Source: CAD feature listing. Evaluate the final solid. Frame: model axes, mm. Face numbers are marked on the shaded views. A direction names the side the tool comes from. Give positions to 0.01 mm unless a question says otherwise; leave off trailing zeros. Order: outer loops, then holes, each group sorted by start corner. A loop starts at its lowest first (then second) coordinate and runs counter-clockwise, first axis right, second up. Notation, with made-up numbers: M -8.75,-6 L 36.25,-6 A23 cw 36.25,19 Z; hole C -13.75,0 d8. An arc over 180 degrees is marked long. Answer in a Markdown table with one row per item. Add a question column.
(1) Section query B-B, the plane y = 22. Return loops of the section in (x, z), plus the area to 3 significant figures.
(2) Material intervals for line 1 along Y through (x, z) = (-11, 23.5); line 2 along Z through (x, y) = (-8, 21); line 3 along X through (y, z) = (9.5, 18.75), sorted ascending.
(3) Section query D-D, the plane x = -13. Return loops of the section in (y, z), plus the area to 3 significant figures.
(4) Set-up query: the marked faces 1, 2, 3 and 4. Return all of +Z, -Z, +X, -X, +Y, -Y with unobstructed straight access to the full face (end or side cutting, diameter ignored); none if empty.
(5) Section query A-A, the plane x = 8. Return loops of the section in (y, z).
(6) Section query C-C, the plane z = 26.25. Return loops of the section in (x, y).
(7) Pin query (flat end, axial travel): P1, Ø2, axis at x = 2, y = 6.5, coming from the -Z side; P2, Ø18, axis at x = 3.5, y = 13.5, coming from the +Z side; P3, Ø3, axis at y = 6.5, z = 14, coming from the +X side; P4, Ø1, axis at y = 30.5, z = 20.5, coming from the +X side. Return the tip coordinate at first contact, or that it passes through.
from build123d import *

# Parameters (mm, degrees)
F1_DEPTH = 15
F3_DEPTH = 28
F0_W     = 23
F0_H     = 10
F4_DEPTH = 15


with BuildPart() as f1:
    # F0 (on Right) → F1 (new body, symmetric)
    with BuildSketch(Plane.YZ):
        Polygon((0, 8), (0, 0), (36, 0), (36, 20), align=None)
    extrude(amount=F1_DEPTH, both=True)

    # F2 (on face) → F3 (join)
    with BuildSketch(Plane(origin=(0, 0, 0), x_dir=(1, 0, 0), z_dir=(0, 0, -1))):
        Polygon((4.5, 0), (-4.5, 0), (-15, -36), (15, -36), align=None)
    extrude(amount=-F3_DEPTH)

    # F0 (on Right) → F4 (cut, symmetric)
    with BuildSketch(Plane.YZ):
        with Locations((11.5, 25)):
            Rectangle(F0_W, F0_H)
    extrude(amount=F4_DEPTH, both=True, mode=Mode.SUBTRACT)


solid = f1.part
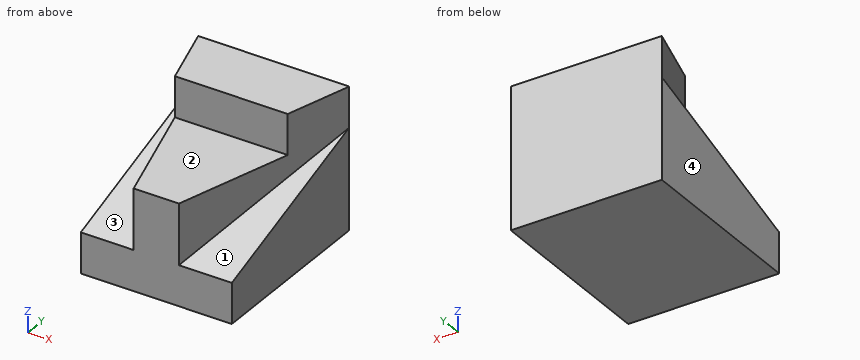
Values follow:
| question | item | result |
|---|---|---|
| 1 | outline | M -15,0 L 15,0 L 15,15.33 L 10.92,15.33 L 10.92,20 L -10.92,20 L -10.92,15.33 L -15,15.33 Z |
| 1 | area | 562 mm² |
| 2 | line 1 | y = 23 to 36 |
| 2 | line 2 | z = 0 to 20 |
| 2 | line 3 | x = -7.27 to 7.27 |
| 3 | outline | M 0,0 L 36,0 L 36,28 L 29.14,28 L 29.14,17.71 L 0,8 Z |
| 3 | area | 567 mm² |
| 4 | face 1 | +Z, +X, -Y |
| 4 | face 2 | +Z, +X, -X, -Y |
| 4 | face 3 | +Z, -X, -Y |
| 4 | face 4 | +Z, -Z, -X, +Y, -Y |
| 5 | outline | M 0,0 L 36,0 L 36,28 L 23,28 L 23,20 L 12,20 L 12,12 L 0,8 Z |
| 6 | outline | M -15,36 L -11.21,23 L 11.21,23 L 15,36 Z |
| 7 | P1 | stops at z = 0 |
| 7 | P2 | stops at z = 20 |
| 7 | P3 | stops at x = 6.83 |
| 7 | P4 | stops at x = 13.54 |
